Read the model definition and answer for the solid it produces. Units are mm, in the model's axes. Face numbers are marked on the shaded views. A direction names the side the tool comes from. Give positions to 0.01 mm unless a question says otherwise; leave off trailing zeros. Write each loop counter-clockwise with the first axis right and the second up, starting at its lowest first coordinate (ties: lowest second). Pieces come first, ordered by that corner, then holes.
```python
from build123d import *

# Parameters (mm, degrees)
SKETCH_9_R                = 19.5
SKETCH_9_R_2              = 2
SKETCH_9_R_3              = 1.5
EXTRUDE_1_DEPTH           = 7.5
EXTRUDE_2_DEPTH           = 12
SKETCH_15_R               = 2
CUT_EXTRUDE_2_DEPTH       = 10.637495374
CUT_EXTRUDE_2_DEPTH_BACK  = 44.637495374
SKETCH_16_R               = 2
CUT_EXTRUDE_3_DEPTH       = 10.637495374
CUT_EXTRUDE_3_DEPTH_BACK  = 44.637495374
SKETCH_17_R               = 2
CUT_EXTRUDE_4_DEPTH       = 3.5
CUT_EXTRUDE_4_DEPTH_BACK  = 37.5
EXTRUDE_3_DEPTH           = 19.5
SKETCH_19_R               = 1.5
SKETCH_19_R_2             = 2
CUT_EXTRUDE_5_DEPTH       = 8.5
CUT_EXTRUDE_5_DEPTH_BACK  = 13
HOLE_WIZARD_3_D           = 3.4
HOLE_WIZARD_3_CSINK_D     = 6.6
HOLE_WIZARD_3_CSINK_ANGLE = 90
CUT_EXTRUDE_6_DEPTH       = 3
CHAMFER_2_SIZE            = 0.5
HOLE_WIZARD_4_D           = 3.2
HOLE_WIZARD_4_CSINK_D     = 6.6
HOLE_WIZARD_4_CSINK_ANGLE = 90


with BuildPart() as part:
    # 草图9 → 凸台-拉伸1 (new body)
    with BuildSketch(Plane(origin=(0, 0, 0), x_dir=(1, 0, 0), z_dir=(0, 1, 0))):
        Circle(SKETCH_9_R)
        with Locations((0, 12.15)):
            Circle(SKETCH_9_R_2, mode=Mode.SUBTRACT)
        with Locations((-10.522208656, -6.075)):
            Circle(SKETCH_9_R_2, mode=Mode.SUBTRACT)
        with Locations((10.522208656, -6.075)):
            Circle(SKETCH_9_R_2, mode=Mode.SUBTRACT)
        with Locations((-11.691342951, 6.75)):
            Circle(SKETCH_9_R_3, mode=Mode.SUBTRACT)
        with Locations((0, -13.5)):
            Circle(SKETCH_9_R_3, mode=Mode.SUBTRACT)
        with Locations((11.691342951, 6.75)):
            Circle(SKETCH_9_R_3, mode=Mode.SUBTRACT)
    extrude(amount=EXTRUDE_1_DEPTH)

    # 草图13 → 凸台-拉伸2 (add)
    with BuildSketch(Plane(origin=(0, 7.5, 0), x_dir=(1, 0, 0), z_dir=(0, 1, 0))):
        with BuildLine():
            Line((-13.7, -11.720210465), (-3.3, -17.724653264))
            ThreePointArc((-3.3, -17.724653264), (0, -18.608885599), (3.3, -17.724653264))
            Line((3.3, -17.724653264), (13.7, -11.720210465))
            ThreePointArc((13.7, -11.720210465), (16.115767665, -9.3044428), (17, -6.0044428))
            Line((17, -6.0044428), (17, 6.0044428))
            ThreePointArc((17, 6.0044428), (16.115767665, 9.3044428), (13.7, 11.720210465))
            Line((13.7, 11.720210465), (3.3, 17.724653264))
            ThreePointArc((3.3, 17.724653264), (0, 18.608885599), (-3.3, 17.724653264))
            Line((-3.3, 17.724653264), (-13.7, 11.720210465))
            ThreePointArc((-13.7, 11.720210465), (-16.115767665, 9.3044428), (-17, 6.0044428))
            Line((-17, 6.0044428), (-17, -6.0044428))
            ThreePointArc((-17, -6.0044428), (-16.115767665, -9.3044428), (-13.7, -11.720210465))
        make_face()
    extrude(amount=EXTRUDE_2_DEPTH)

    # 草图15 → 切除-拉伸2 (cut, two sides)
    with BuildSketch(Plane(origin=(-8.5, 0, -14.722431864), x_dir=(-0.866025404, 0, 0.5), z_dir=(-0.5, 0, -0.866025404))) as cut_extrude_2_sk:
        with Locations((0, 12)):
            Circle(SKETCH_15_R)
    extrude(amount=CUT_EXTRUDE_2_DEPTH, mode=Mode.SUBTRACT)
    extrude(cut_extrude_2_sk.sketch, amount=-CUT_EXTRUDE_2_DEPTH_BACK, mode=Mode.SUBTRACT)

    # 草图16 → 切除-拉伸3 (cut, two sides)
    with BuildSketch(Plane(origin=(8.5, 0, -14.722431864), x_dir=(-0.866025404, 0, -0.5), z_dir=(0.5, 0, -0.866025404))) as cut_extrude_3_sk:
        with Locations((0, 12)):
            Circle(SKETCH_16_R)
    extrude(amount=CUT_EXTRUDE_3_DEPTH, mode=Mode.SUBTRACT)
    extrude(cut_extrude_3_sk.sketch, amount=-CUT_EXTRUDE_3_DEPTH_BACK, mode=Mode.SUBTRACT)

    # 草图17 → 切除-拉伸4 (cut, two sides)
    with BuildSketch(Plane(origin=(17, 0, 0), x_dir=(0, 0, -1), z_dir=(1, 0, 0))) as cut_extrude_4_sk:
        with Locations((0, 12)):
            Circle(SKETCH_17_R)
    extrude(amount=CUT_EXTRUDE_4_DEPTH, mode=Mode.SUBTRACT)
    extrude(cut_extrude_4_sk.sketch, amount=-CUT_EXTRUDE_4_DEPTH_BACK, mode=Mode.SUBTRACT)

    # 草图18 → 凸台-拉伸3 (add)
    with BuildSketch(Plane(origin=(0, 19.5, 0), x_dir=(1, 0, 0), z_dir=(0, 1, 0))):
        Polygon((-7, -4.041451884), (0, -8.082903769), (7, -4.041451884), (7, 4.041451884), (0, 8.082903769), (-7, 4.041451884), align=None)
    extrude(amount=-EXTRUDE_3_DEPTH)

    # 草图19 → 切除-拉伸5 (cut, two sides)
    with BuildSketch(Plane.XZ.offset(-7.5)) as cut_extrude_5_sk:
        with Locations((-11.691342951, -6.75)):
            Circle(SKETCH_19_R)
        with Locations((-10.522208656, 6.075)):
            Circle(SKETCH_19_R_2)
        with Locations((0, 13.5)):
            Circle(SKETCH_19_R)
        with Locations((10.522208656, 6.075)):
            Circle(SKETCH_19_R_2)
        with Locations((11.691342951, -6.75)):
            Circle(SKETCH_19_R)
        with Locations((0, -12.15)):
            Circle(SKETCH_19_R_2)
    extrude(amount=CUT_EXTRUDE_5_DEPTH, mode=Mode.SUBTRACT)
    extrude(cut_extrude_5_sk.sketch, amount=-CUT_EXTRUDE_5_DEPTH_BACK, mode=Mode.SUBTRACT)

    # 打孔尺寸(%根据十字)槽沉头木螺钉的类型3 (through all)
    with Locations(Plane(origin=(0, 19.5, 0), x_dir=(1, 0, 0), z_dir=(0, 1, 0))):
        with Locations((11.691342951, 6.75), (0, -13.5), (-11.691342951, 6.75)):
            CounterSinkHole(HOLE_WIZARD_3_D / 2, HOLE_WIZARD_3_CSINK_D / 2, counter_sink_angle=HOLE_WIZARD_3_CSINK_ANGLE)

    # 草图26 → 切除-拉伸6 (cut)
    with BuildSketch(Plane(origin=(0, 19.5, 0), x_dir=(1, 0, 0), z_dir=(0, 1, 0))):
        with BuildLine():
            Line((17, -6.0044428), (17, 6.0044428))
            ThreePointArc((17, 6.0044428), (16.115767665, 9.3044428), (13.7, 11.720210465))
            Line((13.7, 11.720210465), (3.3, 17.724653264))
            ThreePointArc((3.3, 17.724653264), (0, 18.608885599), (-3.3, 17.724653264))
            Line((-3.3, 17.724653264), (-13.7, 11.720210465))
            ThreePointArc((-13.7, 11.720210465), (-16.115767665, 9.3044428), (-17, 6.0044428))
            Line((-17, 6.0044428), (-17, -6.0044428))
            ThreePointArc((-17, -6.0044428), (-16.115767665, -9.3044428), (-13.7, -11.720210465))
            Line((-13.7, -11.720210465), (-3.3, -17.724653264))
            ThreePointArc((-3.3, -17.724653264), (0, -18.608885599), (3.3, -17.724653264))
            Line((3.3, -17.724653264), (13.7, -11.720210465))
            ThreePointArc((13.7, -11.720210465), (16.115767665, -9.3044428), (17, -6.0044428))
        make_face()
    extrude(amount=-CUT_EXTRUDE_6_DEPTH, mode=Mode.SUBTRACT)

    # 倒角2
    chamfer_2_edges = [part.edges().sort_by_distance(p)[0] for p in [
        (16.115767665, 16.5, 9.3044428),
        (8.5, 16.5, 14.722431864),
        (0, 16.5, 18.608885599),
        (-8.5, 16.5, 14.722431864),
        (-16.115767665, 16.5, 9.3044428),
        (-17, 16.5, 0),
        (-16.115767665, 16.5, -9.3044428),
        (-8.5, 16.5, -14.722431864),
        (0, 16.5, -18.608885599),
        (8.5, 16.5, -14.722431864),
        (16.115767665, 16.5, -9.3044428),
        (17, 16.5, 0),
    ]]
    chamfer(chamfer_2_edges, length=CHAMFER_2_SIZE)

    # 打孔尺寸(%根据十字)槽沉头木螺钉的类型4 (through all)
    with Locations(Plane(origin=(0, 16.5, 0), x_dir=(1, 0, 0), z_dir=(0, 1, 0))):
        with Locations((0, -13.5), (11.691342951, 6.75), (-11.691342951, 6.75)):
            CounterSinkHole(HOLE_WIZARD_4_D / 2, HOLE_WIZARD_4_CSINK_D / 2, counter_sink_angle=HOLE_WIZARD_4_CSINK_ANGLE)


solid = part.part
```
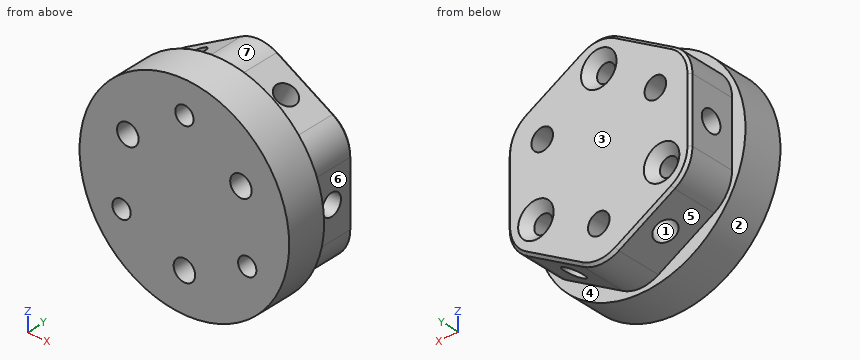
Item 1: Section C-C (y = 5.5) is taken. Write down the section's boundary in (x, z) (3 decimals), and give its area (3 significant figures).
Result set:
outline: circle Ø39 at (0, 0); hole circle Ø3.4 at (-11.691, -6.75); hole circle Ø4 at (-10.522, 6.075); hole circle Ø4 at (0, -12.15); hole circle Ø3.4 at (0, 13.5); hole circle Ø4 at (10.522, 6.075); hole circle Ø3.4 at (11.691, -6.75)
area: 1,130 mm2
Item 2: Find the intervals of material crossed by line 1 along Z through (x, y) = (-1.5, 9); line 2 along X through (y, z) = (13, -9); line 3 along Z through (x, y) = (-12, 12.5), in increasing order.
Result set:
line 1: z = -18.44 to -13.47, -10.83 to 12.7, 14.3 to 18.44
line 2: x = -16.28 to -7.2, -3.2 to 3.2, 7.2 to 16.28
line 3: z = -12.7 to -8.42, -5.08 to -1.94, 1.94 to 4.73, 7.42 to 12.7
Item 3: Which of the six approach directions +Z, -Z, +X, -X, +Y, -Y give full straight-line access (tool end or side, diameter ignored) to the marked faces 4, 5, 6 and 7?
Result set:
face 4: +Y
face 5: -Z, -X, +Y
face 6: +Z, -Z, +X, +Y
face 7: +Z, +Y
Item 4: Section B-B (z = 2.5) is taken. Write down the section's boundary in (x, y).
Result set:
outline: (-19.34, 0) - (19.34, 0) - (19.34, 7.5) - (17, 7.5) - (17, 16) - (16.5, 16.5) - (-16.5, 16.5) - (-17, 16) - (-17, 7.5) - (-19.34, 7.5) - close
Item 5: Section D-D (x = -11.5) is taken. Give the number of separate pieces and of enclosed holes in the cut face, and give its area (3 significant figures).
Result set:
separate pieces: 3
enclosed holes: 1
area: 341 mm2
Item 6: Section A-A (x = 0) is taken. Write down the section's boundary in (y, z), and give its area (3 significant figures).
Result set:
outline: (0, -19.5) - (7.5, -19.5) - (7.5, -18.61) - (16, -18.61) - (16.5, -18.11) - (16.5, -14.15) - (0, -14.15) - close; (0, -10.15) - (16.5, -10.15) - (16.5, 10.2) - (14.9, 11.8) - (0, 11.8) - close; (0, 15.2) - (14.9, 15.2) - (16.5, 16.8) - (16.5, 18.11) - (16, 18.61) - (7.5, 18.61) - (7.5, 19.5) - (0, 19.5) - close
area: 503 mm2
Item 7: Determine the mould class of the marked faces 1, 2 and 3 for opening direction Y: pulls with the +Y half, pulls with the -Y half, needs draft (parallel to the pull), parting line crosses it, or undercut.
Result set:
face 1: undercut
face 2: needs draft
face 3: pulls with the +Y half
Item 8: Each of these flat-tipped pins is pushed along its axis until it touches: pin 1 Ø2.5 at (y, z) = (12, 0) entering from +X; pin 2 Ø4 at (y, z) = (12, -2.5) entering from +X; pin 3 Ø4 at (y, z) = (12.5, -0.5) entering from -X; pin 4 Ø3 at (x, z) = (-11.69, -6.75) entering from -Y. Where does it stop, or does it pass through?
Result set:
pin 1: stops at x = 7
pin 2: stops at x = 17
pin 3: stops at x = -17
pin 4: passes through
